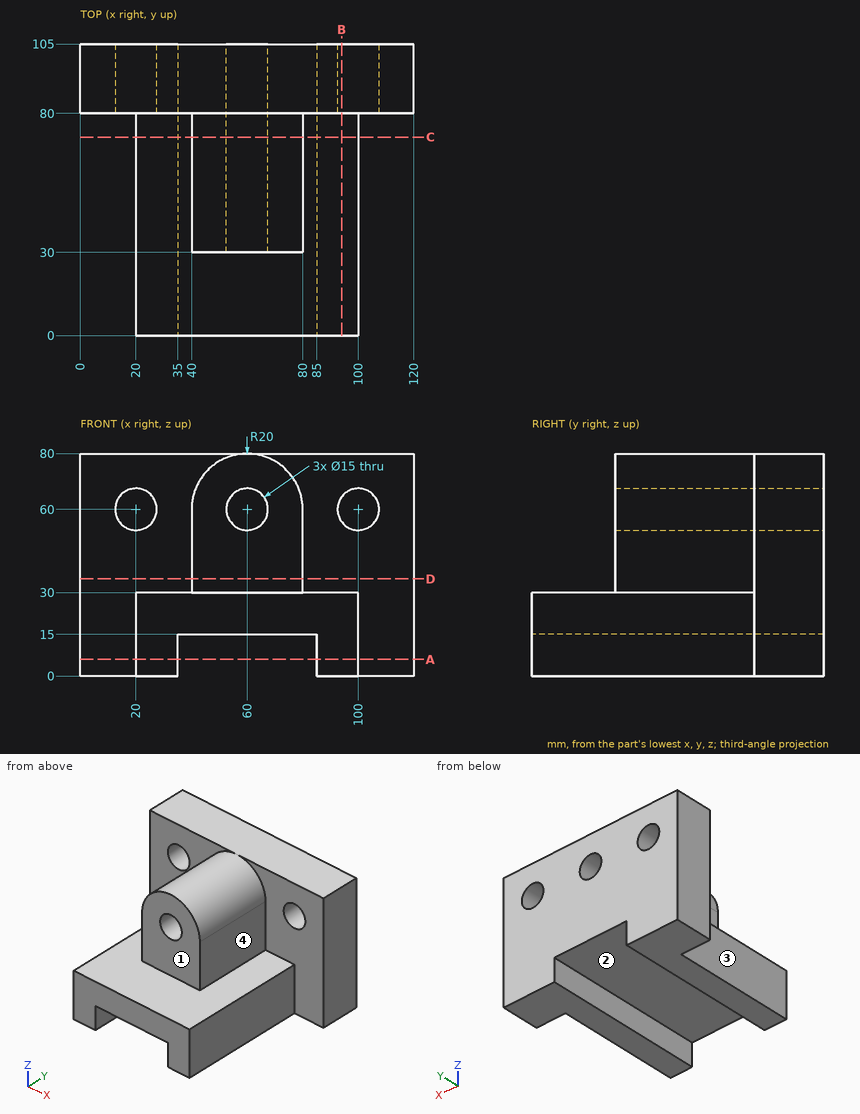
Study the drawing (mm; zero at the part's minimum x, y, z) and answer. A direction names the side the tool comes from. Coordinates: 2 decimals unless noted, no trailing zeros. Write each loop counter-clockwise with the first axis right and the second up, starting at its lowest first coordinate (ties: lowest second). Pieces come first, ordered by that corner, then holes. Notation, with made-up numbers: (54.25, -10.5) - (75.25, -10.5) arc R14 cw to (75.25, -3.5) - close; hole circle Ø7 at (49, 42.25). An arc over 180 degrees is marked (long way). One line per item, written item: value.
1) Find section B-B (x = 94). Give the vertices of the cut face in (y, z), and give its area (4 significant figures).
Geometry check:
outline: (0, 0) - (105, 0) - (105, 55.5) - (80, 55.5) - (80, 30) - (0, 30) - close; (80, 64.5) - (105, 64.5) - (105, 80) - (80, 80) - close
area: 4,175 mm2
2) Find section D-D (z = 35). Give the vertices of the cut face in (x, y), and give its area (3 significant figures).
Geometry check:
outline: (0, 80) - (40, 80) - (40, 30) - (80, 30) - (80, 80) - (120, 80) - (120, 105) - (0, 105) - close
area: 5,000 mm2
3) Find section C-C (y = 71.5). Give the vertices of the cut face in (x, z), and give its area (3 significant figures).
Geometry check:
outline: (20, 0) - (35, 0) - (35, 15) - (85, 15) - (85, 0) - (100, 0) - (100, 30) - (80, 30) - (80, 60) arc R20 ccw to (40, 60) - (40, 30) - (20, 30) - close; hole circle Ø15 at (60, 60)
area: 3,300 mm2
4) A tool of negligible diameter and unlimited length cuts with its end or side. For the marked faces 1, 2, 3 and 4, from which of +Z, -Z, +X, -X, +Y, -Y can it reach the whole face along a straight path? Write none if from no direction.
Geometry check:
face 1: +Z, +X, -X, -Y
face 2: -Z, +Y, -Y
face 3: +Z, -Z, -X, -Y
face 4: +Z, +X, -Y
5) Find section A-A (z = 6). Give the vertices of the cut face in (x, y), and give its area (3 significant figures).
Geometry check:
outline: (0, 80) - (20, 80) - (20, 0) - (35, 0) - (35, 105) - (0, 105) - close; (85, 0) - (100, 0) - (100, 80) - (120, 80) - (120, 105) - (85, 105) - close
area: 4,150 mm2
6) Each of these flat-tipped pins is pushed along its axis until it touches: pin 1 Ø15 at (x, y) = (64, 44.5) entering from -Z; pin 2 Ø24 at (x, z) = (20, 60) entering from -Y; pin 3 Ø8 at (y, z) = (57, 69) entering from -X. Where does it stop, or does it pass through?
Geometry check:
pin 1: stops at z = 15
pin 2: stops at y = 80
pin 3: stops at x = 40.64
7) Consider line 1 along X through (y, z) = (58, 13); line 2 along Z through (x, y) = (60, 65); line 3 along X through (y, z) = (86, 5). Determine where each line is inside the solid, lowest interval first. Write a range as from..to.
Geometry check:
line 1: x = 20..35, 85..100
line 2: z = 15..52.5, 67.5..80
line 3: x = 0..35, 85..120
